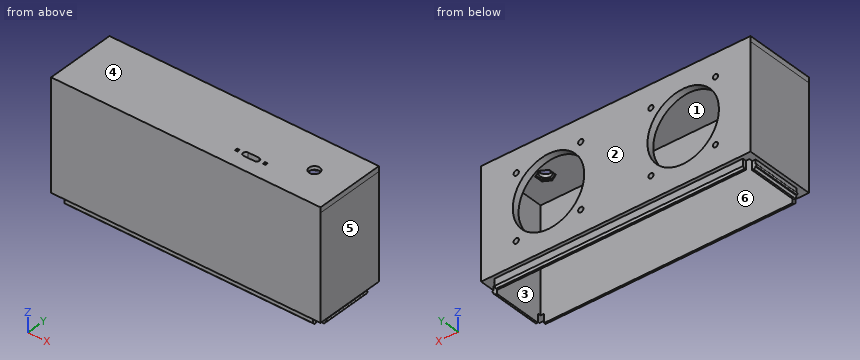
from build123d import *

# Parameters (mm, degrees)
SKETCH021_W     = 150.5
SKETCH021_H     = 36.5
SKETCH021_W_2   = 146.5
SKETCH021_H_2   = 32.5
PAD010_DEPTH    = 5
SKETCH022_W     = 154.5
SKETCH022_H     = 40.5
SKETCH022_W_2   = 146.5
SKETCH022_H_2   = 32.5
PAD011_DEPTH    = 60
SKETCH026_R     = 0.5
PAD013_DEPTH    = 36.5
SKETCH027_W     = 6
SKETCH027_H     = 6
POCKET008_DEPTH = 15
CHAMFER002_SIZE = 1
SKETCH028_W     = 154.5
SKETCH028_H     = 40.5
PAD014_DEPTH    = 3
SKETCH029_R     = 3.1
POCKET009_DEPTH = 5
POCKET010_DEPTH = 1
SKETCH031_W     = 1.5
SKETCH031_H     = 1.5
POCKET011_DEPTH = 5
SKETCH032_R     = 20.5
SKETCH032_R_2   = 1.45
SKETCH032_R_3   = 1.5
POCKET012_DEPTH = 5


with BuildPart() as part:
    # Sketch021 (on DatumPlane) → Pad010 (new body)
    with BuildSketch(Plane.XY.offset(21.399978)):
        with Locations((1.87496, 2.00006)):
            Rectangle(SKETCH021_W, SKETCH021_H)
        with Locations((1.87496, 2.00006)):
            Rectangle(SKETCH021_W_2, SKETCH021_H_2, mode=Mode.SUBTRACT)
    extrude(amount=-PAD010_DEPTH)

    # Sketch022 (on DatumPlane) → Pad011 (join)
    with BuildSketch(Plane.XY.offset(21.399978)):
        with Locations((1.87496, 2.00006)):
            Rectangle(SKETCH022_W, SKETCH022_H)
        with Locations((1.87496, 2.00006)):
            Rectangle(SKETCH022_W_2, SKETCH022_H_2, mode=Mode.SUBTRACT)
    extrude(amount=PAD011_DEPTH)

    # Sketch026 (on Face2 of Pad011) → Pad013 (join)
    with BuildSketch(Plane(origin=(0, 20.25006, 21.399978), x_dir=(-1, 0, 0), z_dir=(0, 1, 0))):
        with Locations((73.375041, -3)):
            Circle(SKETCH026_R)
        with Locations((-77.124959, -3)):
            Circle(SKETCH026_R)
    extrude(amount=-PAD013_DEPTH)

    # Sketch027 (on Face6 of Pad013) → Pocket008 (cut)
    with BuildSketch(Plane(origin=(0, 0, 21.399978), x_dir=(1, 0, 0), z_dir=(0, 0, -1))):
        with Locations((-72.375041, 15.24994)):
            Rectangle(SKETCH027_W, SKETCH027_H)
        with Locations((-72.375041, -19.25006)):
            Rectangle(SKETCH027_W, SKETCH027_H)
        with Locations((76.124959, 15.24994)):
            Rectangle(SKETCH027_W, SKETCH027_H)
        with Locations((76.124959, -19.25006)):
            Rectangle(SKETCH027_W, SKETCH027_H)
    extrude(amount=POCKET008_DEPTH, mode=Mode.SUBTRACT)

    # Chamfer002
    chamfer002_edges = [part.edges().sort_by_distance(p)[0] for p in [
        (1.87496, 20.25006, 16.399978),
        (-73.37504, 2.00006, 16.399978),
        (1.87496, -16.24994, 16.399978),
        (77.12496, 2.00006, 16.399978),
    ]]
    chamfer(chamfer002_edges, length=CHAMFER002_SIZE)

    # Sketch028 (on Face11 of Chamfer002) → Pad014 (join)
    with BuildSketch(Plane.XY.offset(81.399978)):
        with Locations((1.874959, 2.00006)):
            Rectangle(SKETCH028_W, SKETCH028_H)
    extrude(amount=PAD014_DEPTH)

    # Sketch029 (on Face32 of Pad014) → Pocket009 (cut)
    with BuildSketch(Plane.XY.offset(84.399978)):
        with Locations((59.124959, 1.75006)):
            Circle(SKETCH029_R)
    extrude(amount=-POCKET009_DEPTH, mode=Mode.SUBTRACT)

    # Sketch030 (on Face11 of Pocket009) → Pocket010 (cut)
    with BuildSketch(Plane(origin=(0, 0, 81.399978), x_dir=(1, 0, 0), z_dir=(0, 0, -1))):
        Polygon((59.12496, 2.926477), (55.07496, 0.588209), (55.07496, -4.088329), (59.12496, -6.426597), (63.17496, -4.088329), (63.17496, 0.588209), align=None)
    extrude(amount=-POCKET010_DEPTH, mode=Mode.SUBTRACT)

    # Sketch031 (on Face35 of Pocket010) → Pocket011 (cut)
    with BuildSketch(Plane.XY.offset(84.399978)):
        with BuildLine():
            ThreePointArc((28.024959, -6.64994), (26.424959, -8.24994), (28.024959, -9.84994))
            Line((28.024959, -9.84994), (34.224959, -9.84994))
            ThreePointArc((34.224959, -9.84994), (35.824959, -8.24994), (34.224959, -6.64994))
            Line((28.024959, -6.64994), (34.224959, -6.64994))
        make_face()
        with Locations((23.124959, -8.24994)):
            Rectangle(SKETCH031_W, SKETCH031_H)
        with Locations((39.124959, -8.24994)):
            Rectangle(SKETCH031_W, SKETCH031_H)
    extrude(amount=-POCKET011_DEPTH, mode=Mode.SUBTRACT)

    # Sketch032 (on Face13 of Pocket011) → Pocket012 (cut)
    with BuildSketch(Plane(origin=(0, 22.25006, 21.399978), x_dir=(-1, 0, 0), z_dir=(0, 1, 0))):
        with Locations((36.75004, 31.5)):
            Circle(SKETCH032_R)
        with Locations((18.25004, 50)):
            Circle(SKETCH032_R_2)
        with Locations((55.25004, 50)):
            Circle(SKETCH032_R_2)
        with Locations((55.25004, 13)):
            Circle(SKETCH032_R_2)
        with Locations((18.25004, 13)):
            Circle(SKETCH032_R_2)
        with Locations((-40.49996, 31.5)):
            Circle(SKETCH032_R)
        with Locations((-58.99996, 50)):
            Circle(SKETCH032_R_3)
        with Locations((-21.99996, 50)):
            Circle(SKETCH032_R_3)
        with Locations((-21.99996, 13)):
            Circle(SKETCH032_R_3)
        with Locations((-58.99996, 13)):
            Circle(SKETCH032_R_3)
    extrude(amount=-POCKET012_DEPTH, mode=Mode.SUBTRACT)


solid = part.part
Geometry check sheet. Reference: the model listing, model coordinates, mm. Face numbers are marked on the shaded views. A direction names the side the tool comes from. Round coordinates to 2 decimals unless told otherwise and drop trailing zeros. Loops run counter-clockwise (first coordinate to the right, second up) from the corner with the lowest first, then second, coordinate; pieces in that order, holes last.
Item 1: Gauge pin test, flat ends, axial feed: pin 1 (2 mm diameter, centred on x = 5.5, z = 18.5, fed in from -Y); pin 2 (1 mm diameter, centred on x = 50, y = -1.5, fed in from -Z); pin 3 (0.6 mm diameter, centred on y = -3.5, z = 17.5, fed in from -X). Record the tip position at first contact, or that the pin passes through.
Item 2: Thickness scan on line 1 (Y direction, x = 10, z = 42.5); line 2 (X direction, y = -11, z = 71.5); line 3 (X direction, y = 19, z = 65). Record the ranges inside material, lowest first.
Item 3: Access from +Z, -Z, +X, -X, +Y, -Y to the whole of each face (thin tool, end or side, straight path). Record for the marked faces 1 and 2.
Item 4: Cross-section at C-C on x = 12. Record the boundary of the cut face in (y, z), then the cut area to 4 significant figures.
Item 5: Cross-section at D-D on z = 76.5. Record the boundary of the cut face in (x, y), then the cut area to 3 significant figures.
Item 6: Cross-section at A-A on z = 64. Record the boundary of the cut face in (x, y), then the cut area to 3 significant figures.
Item 7: Mould release check, pull along X, two halves, no side actions. Record for the marked faces 3, 4, 5 and 6: pulls with the +X half, pulls with the -X half, needs draft (parallel to the pull), parting line crosses it, or undercut.
Answer sheet:
1. pin 1: stops at y = -16.25
1. pin 2: stops at z = 81.4
1. pin 3: stops at x = -73.38
2. line 1: y = -18.25 to -14.25, 18.25 to 22.25
2. line 2: x = -75.38 to -71.38, 75.12 to 79.12
2. line 3: x = -75.38 to -53.3, -20.2 to 23.95, 57.05 to 79.12
3. face 1: -Z
3. face 2: +Z, -Z, +X, -X, +Y
4. outline: (-18.25, 21.4) - (-16.25, 21.4) - (-16.25, 17.4) - (-15.25, 16.4) - (-14.25, 16.4) - (-14.25, 81.4) - (18.25, 81.4) - (18.25, 16.4) - (19.25, 16.4) - (20.25, 17.4) - (20.25, 21.4) - (22.25, 21.4) - (22.25, 84.4) - (-18.25, 84.4) - close
4. area: 620.5 mm2
5. outline: (-75.38, -18.25) - (79.12, -18.25) - (79.12, 22.25) - (-75.38, 22.25) - close; hole (-71.38, -14.25) - (75.12, -14.25) - (75.12, 18.25) - (-71.38, 18.25) - close
5. area: 1,500 mm2
6. outline: (-75.38, -18.25) - (79.12, -18.25) - (79.12, 22.25) - (57.73, 22.25) - (57.73, 18.25) - (75.12, 18.25) - (75.12, -14.25) - (-71.38, -14.25) - (-71.38, 18.25) - (-53.98, 18.25) - (-53.98, 22.25) - (-75.38, 22.25) - close; (-19.52, 18.25) - (23.27, 18.25) - (23.27, 22.25) - (-19.52, 22.25) - close
6. area: 1,220 mm2
7. face 3: undercut
7. face 4: needs draft
7. face 5: pulls with the +X half
7. face 6: undercut
